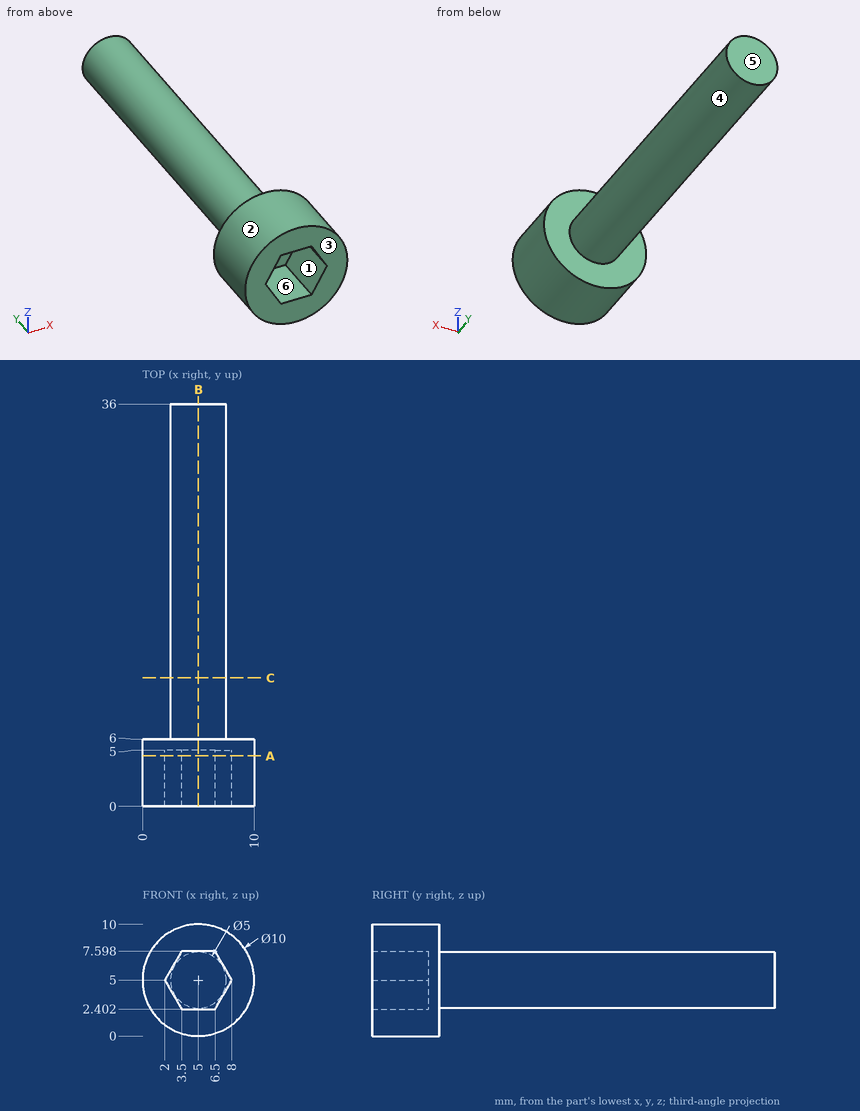
The drawing under review shows one solid part. Ordinate dimensions are in mm from its lowest x, y, z. A direction names the side the tool comes from. Round coordinates to 2 decimals unless told otherwise and drop trailing zeros. Loops run counter-clockwise (first coordinate to the right, second up) from the corner with the lowest first, then second, coordinate; pieces in that order, holes last. Notation, with made-up numbers: (14, -3.5) - (54, -3.5) arc R36 ccw to (54, 32.5) - close; hole circle Ø1 at (32.25, -26). An arc over 180 degrees is marked (long way). One line per item, written item: value. Start each with the question number.
1) Consider section C-C on y = 11.5. Give the boundary of the cut face in (x, z).
2) Consider section A-A on y = 4.5. Give the boundary of the cut face in (x, z).
3) For the marked faces 4, 5 and 6, list the 3-axis set-ups (+Z, -Z, +X, -X, +Y, -Y) from which the entire face can be reached by the end or side of a thin tool; tool diameter is ignored.
4) To check wall thickness, follow L1, parallel to Z at x = 4.75, y = 3.5; L2, parallel to Y at x = 4.75, z = 4.25; L3, parallel to Y at x = 7.25, z = 6.5. State the ranges of each line that lie inside material, in increasing order. Write a range as from..to.
5) Consider section B-B on x = 5. Give the boundary of the cut face in (y, z), then the cut area to 3 significant figures.
6) Insertion check: pin 1 Ø4 at (x, y) = (7.5, 17.5) entering from +Z; pin 2 Ø1.5 at (x, y) = (1.5, 24.5) entering from +Z; pin 3 Ø1 at (y, z) = (4.5, 3.5) entering from +X. Each pin has a flat end and moves straight along its axis. Give the tip position at first contact, or say it passes through.
7) Draft analysis for pull direction Z (two halves, no side actions). For the marked faces 1, 2 and 3, state which applies: +Z half, -Z half, draft (parallel to the pull), parting line (faces both ways), or undercut.
Reported:
1. outline: circle Ø5 at (5, 5)
2. outline: circle Ø10 at (5, 5); hole (2, 5) - (3.5, 2.4) - (6.5, 2.4) - (8, 5) - (6.5, 7.6) - (3.5, 7.6) - close
3. face 4: +Y
3. face 5: +Z, -Z, +X, -X, +Y
3. face 6: -Y
4. L1: z = 0.01..2.4, 7.6..9.99
4. L2: y = 5..36
4. L3: y = 0..6
5. outline: (0, 0) - (6, 0) - (6, 2.5) - (36, 2.5) - (36, 7.5) - (6, 7.5) - (6, 10) - (0, 10) - (0, 7.6) - (5, 7.6) - (5, 2.4) - (0, 2.4) - close
5. area: 184 mm^2
6. pin 1: stops at z = 7.45
6. pin 2: passes through
6. pin 3: stops at x = 9.9
7. face 1: undercut
7. face 2: parting line
7. face 3: draft
